Autodesk Inventor part; units mm, degrees
ref_plane "YZ Plane" through (0, 0, 0) normal (1, 0, 0) x (0, 1, 0)
ref_plane "XZ Plane" through (0, 0, 0) normal (0, 1, 0) x (-1, 0, 0)
ref_plane "XY Plane" through (0, 0, 0) normal (0, 0, 1) x (1, 0, 0)
sketch "草圖1" plane through (0, 0, 0) normal (0, 1, 0) x (-1, 0, 0)
  line L0 (0, 0) -> (5, 0)
  line L1 (5, 0) -> (5, -250)
  line L2 (5, -250) -> (0, -250)
  line L3 (0, -250) -> (0, 0)
  dimension "d0" = 5
  dimension "d1" = 250
extrude "擠出1" add sketch "草圖1" along normal blind 15
sketch "草圖3" plane through (0, 15, 0) normal (0, 1, 0) x (1, 0, 0)
  line L0 (0, 250) -> (-5, 250)
  line L1 (0, 0) -> (-5, 0)
  line L2 (-5, 0) -> (-5, 250)
  line L3 (-5, 250) -> (0, 250)
  line L4 (0, 250) -> (0, 0)
extrude "擠出3" add sketch "草圖3" along normal blind 10
sketch "草圖4" plane through (-5, 0, 0) normal (0, 0, 1) x (1, 0, 0)
  line L0 (5, 0) -> (5, 25)
  line L1 (0, 25) -> (5, 25)
  line L2 (5, 25) -> (0, 25)
  line L3 (5, 25) -> (25, 35)
  line L4 (5, 15) -> (25, 5)
  line L5 (25, 5) -> (25, 35)
  line L6 (0, 0) -> (5, 0)
  line L7 (0, 0) -> (0, 25)
  line L8 (-5, 0) -> (30, 0)
  dimension "d8" = 10
  dimension "d9" = 30
  dimension "d19" = 20
extrude "擠出4" add sketch "草圖4" against normal up to surface (250 mm away) contours L0 L3 L5 L4
shell "薄殼2" thickness 1 removed faces 2 at (20, 15, -83.3333) at (-1.6667, 0, -83.3333)
ref_plane "工作平面1" through (0, 0, -300) normal (0, 0, -1) x (-1, 0, 0)
sketch "草圖5" plane through (0, 0, -300) normal (0, 0, -1) x (-1, 0, 0)
  line L0 (5, 0) -> (0, 0)
  line L1 (0, 0) -> (0, 15)
  line L2 (0, 15) -> (-20, 5)
  line L3 (-20, 5) -> (-20, 35)
  line L4 (-20, 35) -> (0, 25)
  line L5 (5, 25) -> (0, 25)
  line L6 (5, 0) -> (5, 25)
  line L7 (130, -45) -> (-70, -45)
  line L8 (-70, -45) -> (-70, 75)
  line L9 (-70, 75) -> (130, 75)
  line L10 (130, 75) -> (130, -45)
  dimension "d25" = 200
  dimension "d26" = 120
  dimension "d27" = 50
  dimension "d28" = 50
extrude "擠出5" add sketch "草圖5" against normal blind 500
equation "\"d0\" = bottom_w"
equation "\"d1\" = bottom_l"
equation "\"d2\" = bottom_h"
equation "\"d6\" = nuzzle_lh"
equation "\"d8\" = nuzzle_lh"
equation "\"d9\" = 3 * nuzzle_lh"
equation "\"d15\" = nuzzle_lh"
equation "\"bottom_w\" = 5"
equation "\"bottom_l\" = 250"
equation "\"bottom_h\" = 15"
equation "\"nuzzle_lh\" = 10"
properties part number "nuzzle_v1_0310_fluent"
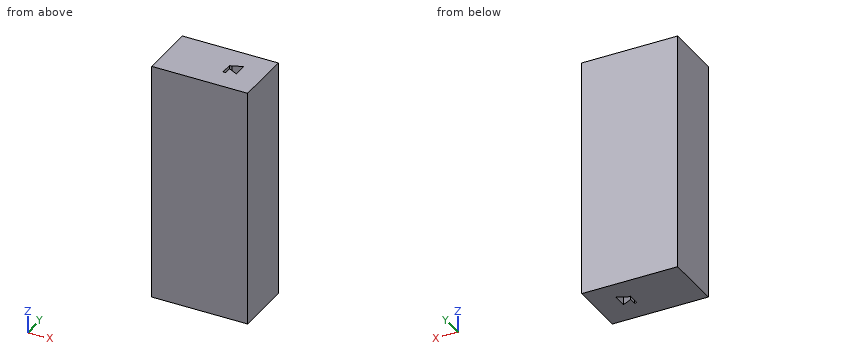
Input: part model. Units: mm. Frame: model coordinates. Coordinates: 2 decimals unless noted, no trailing zeros. Write each loop counter-clockwise with the first axis right and the second up, starting at its lowest first coordinate (ties: lowest second). Pieces come first, ordered by that corner, then holes. Notation, with made-up numbers: M 59.25,33.25 L 96.25,33.25 A16 cw 96.25,54.25 Z; hole C 2.25,45.25 d2. An arc over 180 degrees is marked long. Answer as a JSON object with one key per item and string values. Group by question number.
(1) Section C-C on z = 137.5. Output: boundary loops of the cut face in (x, y), plus the area to 3 significant figures.
(2) Section B-B on x = 11.5. Output: boundary loops of the cut face in (y, z), plus the area to 3 significant figures.
(3) Section A-A on z = -65.5. Output: boundary loops of the cut face in (x, y), plus the area to 3 significant figures.
(4) Ray query, line 1 along Y through (x, z) = (-3, -255.5); line 2 along Y through (x, z) = (-1.5, -227); line 3 along X through (y, z) = (12, -250.5). Return the intervals inside material, ascending. Write a range as [from, to].
Result set:
{
 "1": {"outline": "M -130,-45 L 70,-45 L 70,75 L -130,75 Z; hole M -5,0 L 0,0 L 0,15 L 20,5 L 20,35 L 0,25 L -5,25 Z", "area": "23,500 mm2"},
 "2": {"outline": "M -45,-300 L 9.25,-300 L 9.25,-250 L 30.75,-250 L 30.75,-300 L 75,-300 L 75,200 L 30.75,200 L 30.75,0 L 9.25,0 L 9.25,200 L -45,200 Z; hole M 10.37,-249 L 29.63,-249 L 29.63,-1 L 10.37,-1 Z", "area": "49,800 mm2"},
 "3": {"outline": "M -130,-45 L 70,-45 L 70,75 L -130,75 Z; hole M -4,0 L -1,0 L -1,16.62 L 20,6.12 L 20,33.88 L 0.24,24 L -4,24 Z", "area": "23,600 mm2"},
 "4": {"line 1": "y = [-45, 0], [25, 75]", "line 2": "y = [-45, 0], [24, 75]", "line 3": "x = [-130, -5], [0, 6], [20, 70]"}
}
